```python
from build123d import *

# Parameters (mm, degrees)
BOSS_EXTRUDE1_DEPTH = 25.4
CUT_EXTRUDE1_DEPTH  = 44.994090512
CUT_EXTRUDE2_DEPTH  = 19.05
FILLET1_R           = 2.54
FILLET2_R           = 0.508


with BuildPart() as part:
    # Sketch1 → Boss-Extrude1 (new body)
    with BuildSketch(Plane.XY):
        Polygon((0, 27.94), (0, 12.7), (25.4, 12.7), (25.4, 20.955), align=None)
    extrude(amount=-BOSS_EXTRUDE1_DEPTH)

    # Sketch2 → Cut-Extrude1 (cut, through all)
    with BuildSketch(Plane(origin=(0, 38.1, 0), x_dir=(-1, 0, 0), z_dir=(0, -1, 0))):
        with BuildLine():
            ThreePointArc((-10.414, 12.7), (-11.825185674, 14.811988611), (-14.316446102, 14.316446102))
            Line((-14.316446102, 14.316446102), (-11.083553898, 11.083553898))
            ThreePointArc((-11.083553898, 11.083553898), (-10.588011389, 11.825185674), (-10.414, 12.7))
        make_face()
        with BuildLine():
            Line((-11.083553898, 11.083553898), (-14.316446102, 14.316446102))
            ThreePointArc((-14.316446102, 14.316446102), (-14.316446102, 11.083553898), (-11.083553898, 11.083553898))
        make_face()
    extrude(amount=CUT_EXTRUDE1_DEPTH, mode=Mode.SUBTRACT)

    # Sketch2<3> → Cut-Extrude2 (cut)
    with BuildSketch(Plane(origin=(0, 38.1, 0), x_dir=(-1, 0, 0), z_dir=(0, -1, 0))):
        with BuildLine():
            ThreePointArc((-7.9375, 12.7), (-10.877470153, 17.099976274), (-16.067596045, 16.067596045))
            Line((-16.067596045, 16.067596045), (-14.316446102, 14.316446102))
            ThreePointArc((-14.316446102, 14.316446102), (-11.825185674, 14.811988611), (-10.414, 12.7))
            ThreePointArc((-10.414, 12.7), (-10.588011389, 11.825185674), (-11.083553898, 11.083553898))
            Line((-11.083553898, 11.083553898), (-9.332403955, 9.332403955))
            ThreePointArc((-9.332403955, 9.332403955), (-8.300023726, 10.877470153), (-7.9375, 12.7))
        make_face()
        with BuildLine():
            Line((-14.316446102, 14.316446102), (-16.067596045, 16.067596045))
            ThreePointArc((-16.067596045, 16.067596045), (-16.067596045, 9.332403955), (-9.332403955, 9.332403955))
            Line((-9.332403955, 9.332403955), (-11.083553898, 11.083553898))
            ThreePointArc((-11.083553898, 11.083553898), (-14.316446102, 11.083553898), (-14.316446102, 14.316446102))
        make_face()
    extrude(amount=CUT_EXTRUDE2_DEPTH, mode=Mode.SUBTRACT)

    # Fillet1
    fillet1_edges = [part.edges().sort_by_distance(p)[0] for p in [
        (25.4, 16.8275, -25.4),
        (25.4, 16.8275, 0),
        (0, 20.32, 0),
        (0, 20.32, -25.4),
    ]]
    fillet(fillet1_edges, radius=FILLET1_R)

    # Fillet2
    fillet2_edges = [part.edges().sort_by_distance(p)[0] for p in [
        (12.7, 24.4475, 0),
        (0, 27.94, -12.7),
        (25.4, 20.955, -12.7),
        (12.7, 24.4475, -25.4),
        (24.639618159, 21.164105006, -0.727664709),
        (24.639618159, 21.164105006, -24.672335291),
        (0.760381841, 27.730894994, -24.672335291),
        (0.760381841, 27.730894994, -0.727664709),
    ]]
    fillet(fillet2_edges, radius=FILLET2_R)


solid = part.part
```
The model under review builds one solid part; all positions refer to its coordinate system, in mm. Give positions to 0.01 mm unless a question says otherwise; leave off trailing zeros. Loops run counter-clockwise (first coordinate to the right, second up) from the corner with the lowest first, then second, coordinate; pieces in that order, holes last. Notation, with made-up numbers: (-31.5, 1.5) - (18.5, 1.5) arc R16 cw to (18.5, 5.5) - close; hole circle Ø8 at (62, -40). An arc over 180 degrees is marked (long way). Answer as a JSON object with one key per item and string values.
Q1. To check wall thickness, follow line 1 along Y through (x, z) = (15.75, -13.5); line 2 along Y through (x, z) = (23, -6.5) (3 decimals); line 3 along Z through (x, y) = (16, 22.75). State the ranges of each line that lie inside material, in increasing order.
Worked out:
{"line 1": "y = 12.7 to 19.05", "line 2": "y = 12.7 to 21.615", "line 3": "z = -25.4 to -16.13, -9.27 to 0"}
Q2. Add section B-B on z = -11.5. State the section outline as (x, y) points.
Worked out:
{"outline": "(0, 12.7) - (10.75, 12.7) - (10.75, 19.05) - (8.09, 19.05) - (8.09, 25.71) - (0.64, 27.76) arc R0.51 ccw to (0, 27.27) - close; (14.65, 12.7) - (25.4, 12.7) - (25.4, 20.57) arc R0.51 ccw to (25.03, 21.06) - (17.31, 23.18) - (17.31, 19.05) - (14.65, 19.05) - close"}
Q3. Add section A-A on y = 16.5. State the section outline as (x, z) points.
Worked out:
{"outline": "(0, -22.86) arc R2.54 ccw to (2.54, -25.4) - (22.86, -25.4) arc R2.54 ccw to (25.4, -22.86) - (25.4, -2.54) arc R2.54 ccw to (22.86, 0) - (2.54, 0) arc R2.54 ccw to (0, -2.54) - close; hole circle Ø4.57 at (12.7, -12.7)"}
Q4. Mouldability with a two-part tool opening along Z and no side actions: class faces 1 (the flat face through (15.3, 12.7, -12.5)), 2 (the cylindrical face through (0.724, 19.885, -0.764)), 3 (the flat face through (15, 19.05, -14)), 4 (the cylindrical face through (12.94, 24.23, -25.25)) as +Z half, -Z half, draft (parallel to the pull), parting line (faces both ways), or undercut.
Worked out:
{"face 1": "draft", "face 2": "+Z half", "face 3": "undercut", "face 4": "-Z half"}
Q5. Insertion check: pin 1 (3 mm diameter, centred on x = 14.5, z = -12.5, fed in from +Y); pin 2 (5 mm diameter, centred on x = 8, z = -12.5, fed in from +Y); pin 3 (3 mm diameter, centred on x = 9.5, z = -16, fed in from +Y). Each pin has a flat end and moves straight along its axis. Give the tip position at first contact, or say it passes through.
Worked out:
{"pin 1": "stops at y = 19.05", "pin 2": "stops at y = 26.43", "pin 3": "stops at y = 25.74"}
Q6. Add section C-C on z = -5. State the section outline as (x, y) points.
Worked out:
{"outline": "(0, 12.7) - (25.4, 12.7) - (25.4, 20.57) arc R0.51 ccw to (25.03, 21.06) - (0.64, 27.76) arc R0.51 ccw to (0, 27.27) - close"}
